from build123d import *

# Parameters (mm, degrees)
F0_W     = 1.5875
F0_H     = 3.175
F2_R     = 1.27
F3_SIZE2 = 0.254
F3_SIZE  = 0.508


with BuildPart() as f1:
    # F0 (on Front) → F1 (revolve)
    with BuildSketch(Plane.XZ):
        with Locations((-2.38125, 1.5875)):
            Rectangle(F0_W, F0_H)
    revolve(axis=Axis((0, 0, 3.3253985457), (0, 0, 1)))

    # F2
    f2_edges = [f1.edges().sort_by_distance(p)[0] for p in [
        (3.175, 0, 0),
    ]]
    fillet(f2_edges, radius=F2_R)

    # F3
    f3_edges = [f1.edges().sort_by_distance(p)[0] for p in [
        (1.5875, 0, 0),
    ]]
    f3_side = f1.faces().sort_by_distance((1.5875, 0, 1.5875))[0]
    chamfer(f3_edges, length=F3_SIZE, length2=F3_SIZE2, reference=f3_side)


solid = f1.part
The listing builds one solid part. Answer for the finished solid, in the listing's coordinates (mm). Round coordinates to 2 decimals unless told otherwise and drop trailing zeros. Order: outer loops, then holes, each group sorted by start corner. A loop starts at its lowest first (then second) coordinate and runs counter-clockwise, first axis right, second up. Notation, with made-up numbers: (29.5, 7) -> (81.5, 7) arc R13 cw to (81.5, 21) -> close; hole circle Ø8 at (30.25, 44). An arc over 180 degrees is marked (long way). One line per item, written item: value.
Item 1: Find section D-D, the plane z = 0.7. Give the vertices of the cut face in (x, y) (1 decimal), then the cut area to 3 significant figures.
Taken from the geometry:
outline: circle Ø6.1 at (0, 0); hole circle Ø3.2 at (0, 0)
area: 21.1 mm2
Item 2: Given P1, Ø1, axis at y = 1.5, z = 2.5, coming from the +X side, flat-ended and moving along its own axis, determine where the tip first touches the part or whether it passes through.
Taken from the geometry:
P1: stops at x = 3.01
Item 3: Straight lines are drawn through the part: L1, parallel to X at y = 0, z = 1.55 (1 decimal); L2, parallel to Y at x = 0, z = 1.25; L3, parallel to X at y = -1.25, z = 2.9. For each, find the intervals that lie inside material, in ascending order.
Taken from the geometry:
L1: x = -3.2 to -1.6, 1.6 to 3.2
L2: y = -3.17 to -1.59, 1.59 to 3.17
L3: x = -2.92 to -0.98, 0.98 to 2.92
Item 4: For a pull along X with two mould halves and no side action, classify faces 1 (the cylindrical face through (0.207, -1.574, 1.86)), 2 (the cylindrical face through (0.69, 3.1, 2.24)), 3 (the flat face through (-1.4, 1.4, 3.175)) as released by +X, released by -X, zero draft, split by the parting line, or undercut.
Taken from the geometry:
face 1: undercut
face 2: split by the parting line
face 3: zero draft
